Geometry check sheet. Reference: the model listing, model coordinates, mm. Face numbers are marked on the shaded views. Give positions to 0.01 mm unless a question says otherwise; leave off trailing zeros. Write each loop counter-clockwise with the first axis right and the second up, starting at its lowest first coordinate (ties: lowest second). Pieces come first, ordered by that corner, then holes. Notation, with made-up numbers: (26, 52) -> (56, 52) arc R20 ccw to (56, 60) -> close; hole circle Ø5 at (39, 71). An arc over 180 degrees is marked (long way). Write item = value, one per line. Start each with the question number.
1. Mould release check, pull along X, two halves, no side actions. Record for the marked faces 1, 2, 3 and 4: pulls with the +X half, pulls with the -X half, needs draft (parallel to the pull), parting line crosses it, or undercut.
2. Cross-section at C-C, the plane y = -36.5. Record the cut outline in (x, z), plus the area to 3 significant figures.
3. Cross-section at A-A, the plane z = 4.75. Record the cut outline in (x, y).
4. Thickness scan on line 1 along Y through (x, z) = (64, -5.25); line 2 along X through (y, z) = (-161, -3.5); line 3 along Z through (x, y) = (68, -147). Record the ranges inside material, lowest first.
5. Cross-section at B-B, the plane x = 97. Record the cut outline in (y, z), plus the area to 3 significant figures.
6. Depth check by flat-ended pin: P1, Ø1.6, axis at x = -3, y = -1, coming from the +Z side; P2, Ø6, axis at x = -74.5, y = -41, coming from the +Z side. Enter the tip coordinate at first touch or a pass-through.
```python
from build123d import *

# Parameters (mm, degrees)
F1_DEPTH = 190
F2_W     = 230
F2_H     = 20
F3_DEPTH = 2
F6_DEPTH = 190.001


# Not quite as in the source:
# - a pattern or mirror of a feature is missing from the dataset's text; its kind, count and spacing are read off the source's solid


with BuildPart() as f1:
    # F0 (on Front) → F1 (new body)
    with BuildSketch(Plane.XZ):
        Polygon((-115, 10), (-115, -10), (115, -10), (115, 10), (113, 10), (113, -8), (-113, -8), (-113, 10), align=None)
    extrude(amount=F1_DEPTH)

    # F2 (on face) → F3 (join)
    with BuildSketch(Plane.XZ.offset(190)):
        Rectangle(F2_W, F2_H)
    f3 = extrude(amount=-F3_DEPTH)

    # F3_copies: F3 across plane
    add(f3.mirror(Plane.ZX.offset(-95)))

    # F5 (on face) → F6 (cut, through all)
    with BuildSketch(Plane.XZ.offset(190)):
        Polygon((-20, 0), (0, 0), (20, 0), (30, 10), (0, 10), (-30, 10), align=None)
    extrude(amount=-F6_DEPTH, mode=Mode.SUBTRACT)


solid = f1.part
```
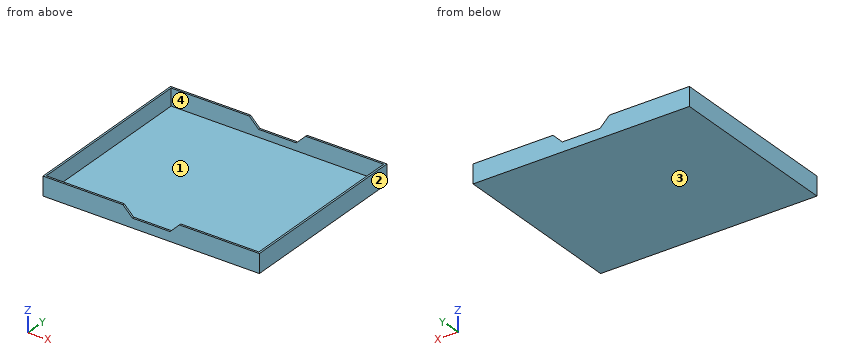
Answers:
q1.face_1 = undercut
q1.face_2 = pulls with the +X half
q1.face_3 = needs draft
q1.face_4 = undercut
q2.outline = (-115, -10) -> (115, -10) -> (115, 10) -> (113, 10) -> (113, -8) -> (-113, -8) -> (-113, 10) -> (-115, 10) -> close
q2.area = 532 mm^2
q3.outline = (-115, -190) -> (-24.75, -190) -> (-24.75, -188) -> (-113, -188) -> (-113, -2) -> (-24.75, -2) -> (-24.75, 0) -> (-115, 0) -> close; (24.75, -190) -> (115, -190) -> (115, 0) -> (24.75, 0) -> (24.75, -2) -> (113, -2) -> (113, -188) -> (24.75, -188) -> close
q4.line_1 = -190 to -188, -2 to 0
q4.line_2 = -115 to -113, 113 to 115
q4.line_3 = -10 to -8
q5.outline = (-190, -10) -> (0, -10) -> (0, 10) -> (-2, 10) -> (-2, -8) -> (-188, -8) -> (-188, 10) -> (-190, 10) -> close
q5.area = 452 mm^2
q6.P1 = 0
q6.P2 = -8
